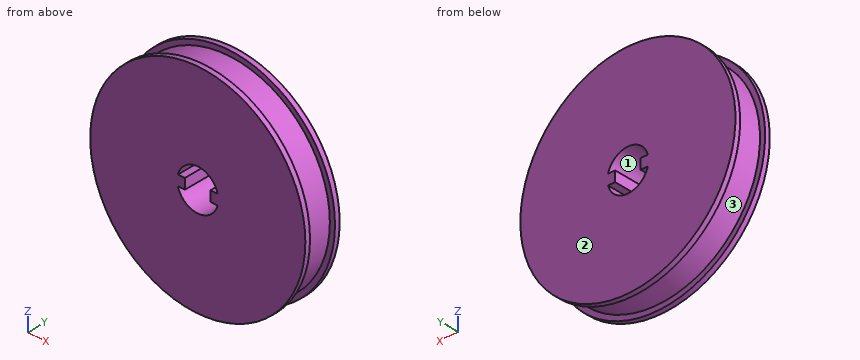
from build123d import *

# Parameters (mm, degrees)
ESQUISSE6_W        = 4.5
ESQUISSE6_H        = 3
BOSS_EXTRU_1_DEPTH = 11


with BuildPart() as part:
    # Esquisse2 → Révolution1 (revolve)
    with BuildSketch(Plane.XY):
        Polygon((6, 5.365286165), (6, -5.634713835), (31.5, -5.634713835), (31.5, -4.134713835), (30, -4.134713835), (30, 3.865286165), (31.5, 3.865286165), (31.5, 5.365286165), align=None)
    revolve(axis=Axis((0, 0, 0), (0, 1, 0)))

    # Esquisse6 → Boss.-Extru.1 (add)
    with BuildSketch(Plane(origin=(0, 5.365286165, 0), x_dir=(1, 0, 0), z_dir=(0, 1, 0))):
        with Locations((-6, 0)):
            Rectangle(ESQUISSE6_W, ESQUISSE6_H)
        with Locations((6, 0)):
            Rectangle(ESQUISSE6_W, ESQUISSE6_H)
    extrude(amount=-BOSS_EXTRU_1_DEPTH)


solid = part.part
Part model, mm, in its own coordinate system. Face numbers are marked on the shaded views. Give positions to 0.01 mm unless a question says otherwise; leave off trailing zeros. Order: outer loops, then holes, each group sorted by start corner. A loop starts at its lowest first (then second) coordinate and runs counter-clockwise, first axis right, second up. Notation, with made-up numbers: (61.5, 60) -> (73.5, 60) arc R19 ccw to (73.5, 73) -> close; hole circle Ø5 at (34, 60.25). An arc over 180 degrees is marked (long way). Use one line per item in the form item = value.
(1) Saw through at C-C (z = 0). Write the cut outline in (x, y).
Solution:
outline = (-31.5, -5.63) -> (-3.75, -5.63) -> (-3.75, 5.37) -> (-31.5, 5.37) -> (-31.5, 3.87) -> (-30, 3.87) -> (-30, -4.13) -> (-31.5, -4.13) -> close; (3.75, -5.63) -> (31.5, -5.63) -> (31.5, -4.13) -> (30, -4.13) -> (30, 3.87) -> (31.5, 3.87) -> (31.5, 5.37) -> (3.75, 5.37) -> close
(2) Pull direction Z, two halves, no side cores. Call the marked faces 1, 2 and 3: +Z half, -Z half, draft (parallel to the pull), parting line (faces both ways), or undercut.
Solution:
face_1 = undercut
face_2 = draft
face_3 = parting line
(3) Drill centre lines: line 1 (Z direction, x = -4.5, y = 3); line 2 (Y direction, x = 16, z = 27); line 3 (Z direction, x = -5, y = -3.25). Where is each one in solid material? Low to high. Write a range as from..to.
Solution:
line_1 = -29.66..-3.97, -1.5..1.5, 3.97..29.66
line_2 = -5.63..-4.13, 3.87..5.37
line_3 = -29.58..-3.32, -1.5..1.5, 3.32..29.58
(4) Flat gauge pins, fed straight in: P1, Ø0.9, axis at y = 0, z = -0.5, coming from the +X side; P2, Ø3, axis at y = -0.5, z = 20.5, coming from the -X side; P3, Ø2, axis at y = 0.5, z = -10, coming from the -X side. Where does each tip first touch, or does it go through?
Solution:
P1 = 30
P2 = -23.22
P3 = -28.62
(5) Saw through at D-D (z = 27.5). Write the cut outline in (x, y), then the cut area to 3 significant figures.
Solution:
outline = (-15.36, -5.63) -> (15.36, -5.63) -> (15.36, -4.13) -> (11.99, -4.13) -> (11.99, 3.87) -> (15.36, 3.87) -> (15.36, 5.37) -> (-15.36, 5.37) -> (-15.36, 3.87) -> (-11.99, 3.87) -> (-11.99, -4.13) -> (-15.36, -4.13) -> close
area = 284 mm²
(6) Saw through at A-A (x = 0). Write the cut outline in (y, z), then the cut area to 3 significant figures.
Solution:
outline = (-5.63, -31.5) -> (-4.13, -31.5) -> (-4.13, -30) -> (3.87, -30) -> (3.87, -31.5) -> (5.37, -31.5) -> (5.37, -6) -> (-5.63, -6) -> close; (-5.63, 6) -> (5.37, 6) -> (5.37, 31.5) -> (3.87, 31.5) -> (3.87, 30) -> (-4.13, 30) -> (-4.13, 31.5) -> (-5.63, 31.5) -> close
area = 537 mm²
(7) Saw through at B-B (y = 1.5). Write the cut outline in (x, z).
Solution:
outline = circle Ø60 at (0, 0); hole (-5.81, -1.5) arc R6 ccw to (5.81, -1.5) -> (3.75, -1.5) -> (3.75, 1.5) -> (5.81, 1.5) arc R6 ccw to (-5.81, 1.5) -> (-3.75, 1.5) -> (-3.75, -1.5) -> close
